Check sheet for the modelled part. Datum: model origin and axes. Units: mm. Face numbers are marked on the shaded views. Round coordinates to 2 decimals unless told otherwise and drop trailing zeros. Write each loop counter-clockwise with the first axis right and the second up, starting at its lowest first coordinate (ties: lowest second). Pieces come first, ordered by that corner, then holes. Notation, with made-up numbers: (64, 14) -> (116, 14) arc R16 ccw to (116, 41) -> close; hole circle Ø1 at (-30, 76.25). An arc over 180 degrees is marked (long way). One line per item, written item: value.
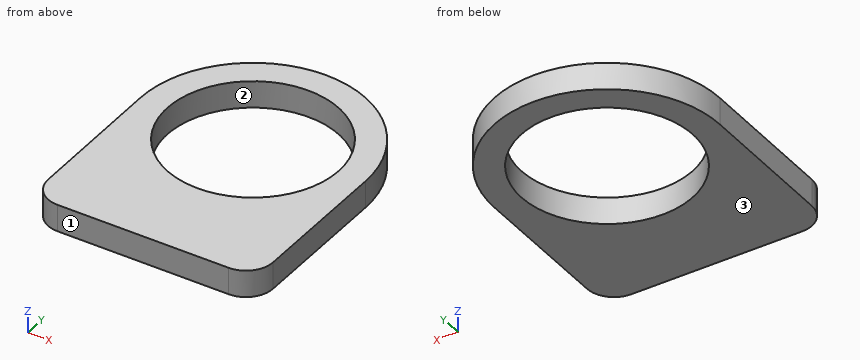
from build123d import *

# Parameters (mm, degrees)
F0_R     = 15.841056
F1_DEPTH = 5


with BuildPart() as f1:
    # F0 (on Top) → F1 (new body)
    with BuildSketch(Plane.XY):
        with BuildLine():
            Line((20.728503, -26.431861), (20.840867, -0.088895))
            ThreePointArc((20.840867, -0.088895), (0.044448, 20.841009), (-20.841056, 0))
            Line((-20.841056, 0), (-20.841056, -26.410534))
            ThreePointArc((-20.841056, -26.410534), (-19.37659, -29.946068), (-15.841056, -31.410534))
            Line((-15.841056, -31.410534), (15.728548, -31.410534))
            ThreePointArc((15.728548, -31.410534), (19.256534, -29.9536), (20.728503, -26.431861))
        make_face()
        Circle(F0_R, mode=Mode.SUBTRACT)
    extrude(amount=F1_DEPTH)


solid = f1.part
Item 1: Sectioned sample at B-B (z = 2.15). Enter the section's corners in (x, y).
Result set:
outline: (-20.84, -26.41) arc R5 ccw to (-15.84, -31.41) -> (15.73, -31.41) arc R5 ccw to (20.73, -26.43) -> (20.84, -0.09) arc R20.84 ccw to (-20.84, 0) -> close; hole circle Ø31.68 at (0, 0)
Item 2: Release check for a two-part mould opening along Y. For the marked faces 1, 2 and 3 record: pulls with the +Y half, pulls with the -Y half, needs draft (parallel to the pull), parting line crosses it, or undercut.
Result set:
face 1: pulls with the -Y half
face 2: undercut
face 3: needs draft
Item 3: Sectioned sample at C-C (y = -7). Enter the section's corners in (x, z).
Result set:
outline: (-20.84, 0) -> (-14.21, 0) -> (-14.21, 5) -> (-20.84, 5) -> close; (14.21, 0) -> (20.81, 0) -> (20.81, 5) -> (14.21, 5) -> close
Item 4: Depth check by flat-ended pin: pin 1 (2 mm diameter, centred on y = 6.5, z = 3, fed in from -X); pin 2 (1.5 mm diameter, centred on y = 1.5, z = 4, fed in from +X). Enter the tip coordinate at first touch or a pass-through.
Result set:
pin 1: x = -20.1
pin 2: x = 20.83
Item 5: Material ranges on line 1 along Y through (x, z) = (-0.5, 1.15); line 2 along X through (y, z) = (-1.5, 0.9); line 3 along X through (y, z) = (-8.5, 2.95) (3 decimals), recorded low to high.
Result set:
line 1: -31.41 to -15.83, 15.83 to 20.84
line 2: -20.84 to -15.77, 15.77 to 20.83
line 3: -20.841 to -13.367, 13.367 to 20.805
Item 6: Sectioned sample at A-A (x = 0). Enter the section's corners in (y, z), then the cut area to 3 significant figures.
Result set:
outline: (-31.41, 0) -> (-15.84, 0) -> (-15.84, 5) -> (-31.41, 5) -> close; (15.84, 0) -> (20.84, 0) -> (20.84, 5) -> (15.84, 5) -> close
area: 103 mm^2
